Here's how the part is built. I have some questions about the finished solid (model axes, mm). A direction names the side the tool comes from. Give positions to 0.01 mm unless a question says otherwise; leave off trailing zeros. Write each loop counter-clockwise with the first axis right and the second up, starting at its lowest first coordinate (ties: lowest second). Pieces come first, ordered by that corner, then holes. Notation, with made-up numbers: (-12.75, 75.25) - (-8.75, 75.25) arc R10 ccw to (-8.75, 81.25) - close; hole circle Ø10 at (62.5, -25.5). An arc over 180 degrees is marked (long way). Write each question's results on one line, items separated by ' | '. Start each with the question number.
Item 1: Will these pins go through, and if not, where does the flat tip stop? P1, Ø11.5, axis at x = 0, y = 2.5, coming from the -Z side; P2, Ø3, axis at x = 2.5, y = 27.5, coming from the +Z side; P3, Ø3, axis at y = 29.5, z = 4.5, coming from the -X side; P4, Ø5.5, axis at x = -0.5, z = -9.5, coming from the -Y side.
Item 2: Please list where these lines run through material, in increasing order: line 1 along Y through (x, z) = (13.9, 0.8); line 2 along Z through (x, y) = (7.5, 27.5); line 3 along Y through (x, z) = (-2.5, 5).
Item 3: Which directions (+Z, -Z, +X, -X, +Y, -Y) give clear straight access to the entire face, cutting with the end or side of a thin tool? Please do faces 4 (the flat face through (0, 28, -6.35)), 5 (the flat face through (3, 28, 4)), 6 (the flat face through (-4.3, 30, 4)), 7 (the flat face through (2.3, 30, 4)), 8 (the flat face through (4.3, 30, 4)).
Item 4: We'd pull the mould along X, two halves only. Please class faces 1 (the flat face through (-3, 30, 7)), 2 (the flat face through (19, 10.3, 0.3)), 3 (the cylindrical face through (12.79, -22.24, 1.01)): +X half, -X half, draft (parallel to the pull), parting line (faces both ways), or undercut.
Item 5: Suppose I cut it at B-B on z = 3. List the corners of the cut face in (x, y) for me.
Item 6: Suppose I cut it at C-C on y = -23.25. List the corners of the cut face in (x, z) for me.
Item 7: Suppose I cut it at A-A on x = -13.9. List the corners of the cut face in (y, z) for me, then the cut area to 3 significant figures.
Item 8: Suppose I cut it at D-D on x = 7. List the corners of the cut face in (y, z) for me.
```python
from build123d import *

# Parameters (mm, degrees)
F0_W     = 38
F0_H     = 60
F1_DEPTH = 2
F2_W     = 38
F2_H     = 2
F2_H_2   = 6.35
F3_DEPTH = 2
F4_W     = 38
F4_H     = 6
F5_DEPTH = 5
F6_W     = 2
F6_H     = 4
F7_DEPTH = 5
F8_R     = 1.5
F9_DEPTH = 25


with BuildPart() as f1:
    # F0 (on Top) → F1 (new body)
    with BuildSketch(Plane.XY):
        Rectangle(F0_W, F0_H)
    extrude(amount=F1_DEPTH)

    # F2 (on face) → F3 (join)
    with BuildSketch(Plane(origin=(0, 30, 0), x_dir=(-1, 0, 0), z_dir=(0, 1, 0))):
        with Locations((0, 1)):
            Rectangle(F2_W, F2_H)
        with Locations((0, -3.175)):
            Rectangle(F2_W, F2_H_2)
    extrude(amount=F3_DEPTH)

    # F4 (on face) → F5 (join)
    with BuildSketch(Plane(origin=(0, 0, -6.35), x_dir=(1, 0, 0), z_dir=(0, 0, -1))):
        with Locations((0, -29)):
            Rectangle(F4_W, F4_H)
    extrude(amount=F5_DEPTH)

    # F6 (on face) → F7 (join)
    with BuildSketch(Plane.XY.offset(2)):
        with Locations((-3.3, 30)):
            Rectangle(F6_W, F6_H)
        with Locations((3.3, 30)):
            Rectangle(F6_W, F6_H)
    extrude(amount=F7_DEPTH)

    # F8 (on face) → F9 (cut)
    with BuildSketch(Plane.XY.offset(2)):
        with Locations((-13.9, -23.25)):
            Circle(F8_R)
        with Locations((13.9, -23.25)):
            Circle(F8_R)
    extrude(amount=-F9_DEPTH, mode=Mode.SUBTRACT)


solid = f1.part
```
Checked values:
1) P1: stops at z = 0 | P2: stops at z = 7 | P3: stops at x = -4.3 | P4: stops at y = 26
2) line 1: y = -30 to -24.75, -21.75 to 32 | line 2: z = -11.35 to -6.35, 0 to 2 | line 3: y = 28 to 32
3) face 4: +X, -X, -Y | face 5: +Z, +X, -X, -Y | face 6: +Z, -X, +Y, -Y | face 7: +Z, +Y, -Y | face 8: +Z, +X, +Y, -Y
4) face 1: draft | face 2: +X half | face 3: undercut
5) outline: (-4.3, 28) - (-2.3, 28) - (-2.3, 32) - (-4.3, 32) - close; (2.3, 28) - (4.3, 28) - (4.3, 32) - (2.3, 32) - close
6) outline: (-19, 0) - (-15.4, 0) - (-15.4, 2) - (-19, 2) - close; (-12.4, 0) - (12.4, 0) - (12.4, 2) - (-12.4, 2) - close; (15.4, 0) - (19, 0) - (19, 2) - (15.4, 2) - close
7) outline: (-30, 0) - (-24.75, 0) - (-24.75, 2) - (-30, 2) - close; (-21.75, 0) - (30, 0) - (30, -6.35) - (26, -6.35) - (26, -11.35) - (32, -11.35) - (32, 2) - (-21.75, 2) - close | area: 161 mm^2
8) outline: (-30, 0) - (30, 0) - (30, -6.35) - (26, -6.35) - (26, -11.35) - (32, -11.35) - (32, 2) - (-30, 2) - close
